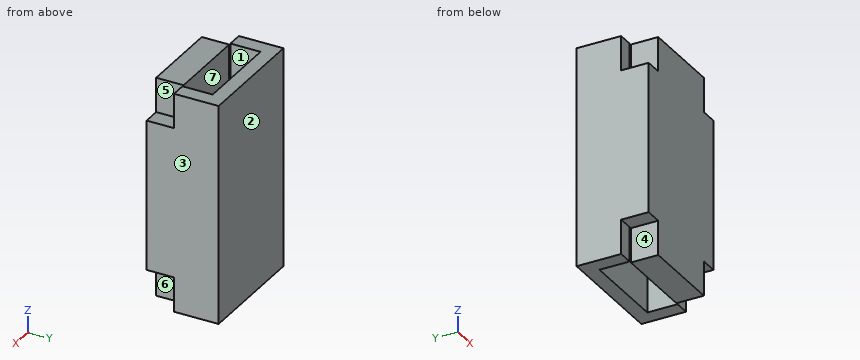
```python
from build123d import *

# Parameters (mm, degrees)
SKETCH1_W           = 13.525
SKETCH1_H           = 7.40621
SKETCH1_W_2         = 10
SKETCH1_H_2         = 3.5
BOSS_EXTRUDE1_DEPTH = 12.7
SKETCH2_W           = 2
SKETCH2_H           = 3.175
SKETCH2_W_2         = 13.525
SKETCH2_H_2         = 0.939
CUT_EXTRUDE2_DEPTH  = 4
SKETCH2_4_W         = 13.525
SKETCH2_4_H         = 0.939
BOSS_EXTRUDE2_DEPTH = 12.7


with BuildPart() as part:
    # Sketch1 → Boss-Extrude1 (new body, symmetric)
    with BuildSketch(Plane.XY):
        with Locations((0, -1.221895)):
            Rectangle(SKETCH1_W, SKETCH1_H)
        Rectangle(SKETCH1_W_2, SKETCH1_H_2, mode=Mode.SUBTRACT)
    extrude(amount=BOSS_EXTRUDE1_DEPTH, both=True)

    # Sketch2 → Cut-Extrude2 (cut)
    with BuildSketch(Plane.XY.offset(12.7)):
        with Locations((-5.7625, -3.3375)):
            Rectangle(SKETCH2_W, SKETCH2_H)
        with Locations((5.7625, -3.3375)):
            Rectangle(SKETCH2_W, SKETCH2_H)
        with Locations((0, 2.95071)):
            Rectangle(SKETCH2_W_2, SKETCH2_H_2)
    cut_extrude2 = extrude(amount=-CUT_EXTRUDE2_DEPTH, mode=Mode.SUBTRACT)

    # Sketch2_4 → Boss-Extrude2 (add)
    with BuildSketch(Plane.XY.offset(12.7)):
        with Locations((0, 2.95071)):
            Rectangle(SKETCH2_4_W, SKETCH2_4_H)
    boss_extrude2 = extrude(amount=-BOSS_EXTRUDE2_DEPTH)

    # Mirror1: Cut-Extrude2, Boss-Extrude2 across plane
    add(cut_extrude2.mirror(Plane.XY), mode=Mode.SUBTRACT)
    add(boss_extrude2.mirror(Plane.XY))


solid = part.part
```
Design review of the part built by this model. Coordinates are the model's own, in mm. Face numbers are marked on the shaded views. A direction names the side the tool comes from. Coordinates: 2 decimals unless noted, no trailing zeros. Loops run counter-clockwise (first coordinate to the right, second up) from the corner with the lowest first, then second, coordinate; pieces in that order, holes last. Notation, with made-up numbers: M 49,-26.5 L 73,-26.5 A18 cw 73,-22.5 Z; hole C 89.25,43 d11. An arc over 180 degrees is marked long. One line per question, with ' | ' between items.
(1) Wall thickness on probe 1 along Y at (x, z) = (0.5, -4) (3 decimals); probe 2 along X at (y, z) = (1, -5.75); probe 3 along Y at (x, z) = (6, 9): over which ranges is each line inside the solid? List them lowest first.
Filled in:
probe 1: y = -4.925 to -1.75, 1.75 to 3.42 | probe 2: x = -6.76 to -5, 5 to 6.76 | probe 3: y = -1.75 to 3.42
(2) We need section D-D (x = -4.5). Give the boundary of the cut face in (y, z) (3 decimals), and give its area (3 significant figures).
Filled in:
outline: M -4.925,-12.7 L -1.75,-12.7 L -1.75,12.7 L -4.925,12.7 Z; M 1.75,-12.7 L 3.42,-12.7 L 3.42,12.7 L 1.75,12.7 Z | area: 123 mm^2
(3) Machinability: for the marked faces 4, 5, 6 and 7, which of the approach directions +Z, -Z, +X, -X, +Y, -Y give a long, thin tool a straight path to every point of the face, cutting with its end or side? Answer none if there is none.
Filled in:
face 4: -Z, -X, -Y | face 5: +Z, +X, -Y | face 6: -Z, +X, -Y | face 7: +Z, -Z
(4) For pin 1 Ø0.5 at (x, z) = (5.5, 10) entering from -Y; pin 2 Ø1.6 at (y, z) = (-3.5, -10.5) entering from -X; pin 3 Ø1 at (x, y) = (6, -4) entering from +Z; pin 4 Ø1 at (x, y) = (-2, 1) entering from +Z, all flat-tipped, find the tip position at first contact; note any pin that passes through.
Filled in:
pin 1: stops at y = -1.75 | pin 2: stops at x = -4.76 | pin 3: stops at z = 8.7 | pin 4: passes through
(5) We need section B-B (y = 0.5). Give the boundary of the cut face in (x, z).
Filled in:
outline: M -6.76,-12.7 L -5,-12.7 L -5,12.7 L -6.76,12.7 Z; M 5,-12.7 L 6.76,-12.7 L 6.76,12.7 L 5,12.7 Z
(6) Draft analysis for pull direction X (two halves, no side actions). For the marked faces 1, 2 and 3, state which applies: released by +X, released by -X, zero draft, split by the parting line, or undercut.
Filled in:
face 1: undercut | face 2: zero draft | face 3: released by +X
